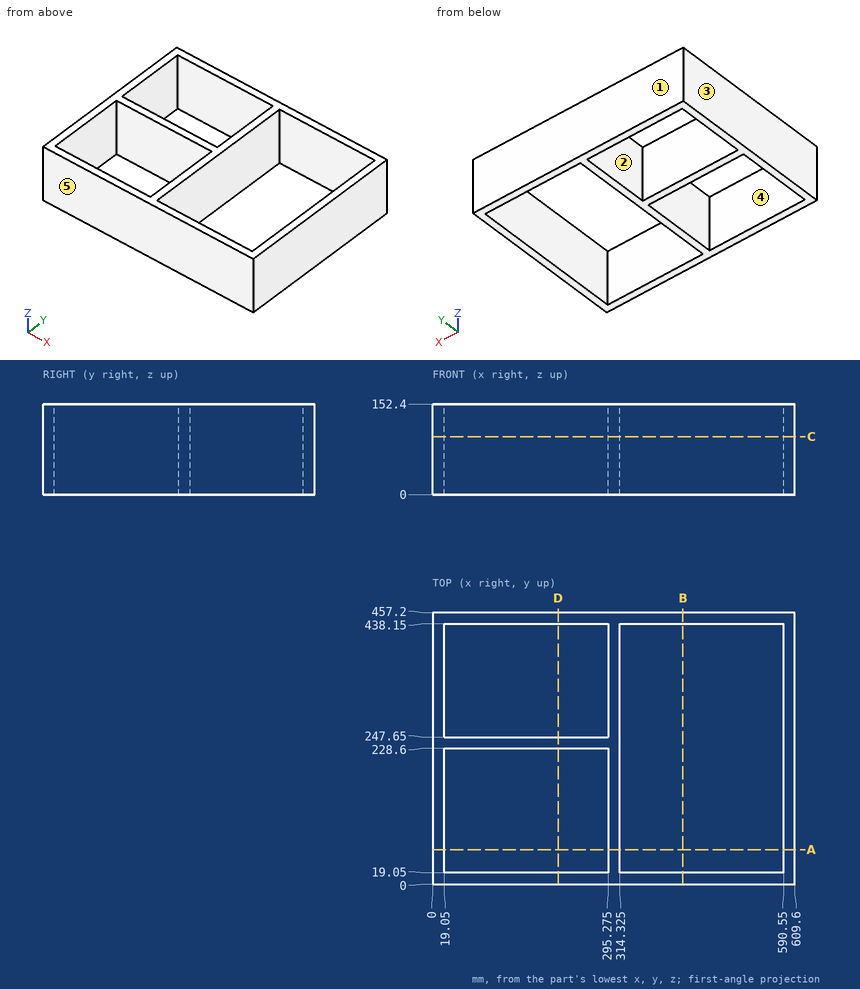
Answer from the drawing. Dimensions are ordinates in mm from the lowest x, y and z of the part. A direction names the side the tool comes from. Give positions to 0.01 mm unless a question says otherwise; leave off trailing zeros. Loops run counter-clockwise (first coordinate to the right, second up) from the corner with the lowest first, then second, coordinate; pieces in that order, holes last. Notation, with made-up numbers: (70, 68.25) - (108, 68.25) arc R24 ccw to (108, 78.25) - close; hole circle Ø9 at (30.25, -24.75). An arc over 180 degrees is marked (long way). Answer as CSV lines item,"result". Start each with the question number.
Item 1: Find the intervals of material crossed by line 1 (X direction, y = 334, z = 71.5) (3 decimals); line 2 (Y direction, x = 234.5, z = 42.5), in increasing order. Write a range as from..to.
Item 2: The mould has two halves that part along Y. Classify the marked faces 1, 2 and 3: +Y half, -Y half, draft (parallel to the pull), parting line (faces both ways), or undercut.
Item 3: A cutting plane is placed at B-B on x = 421. Determine the outline of the cut face in (y, z), then the cut area to 3 significant figures.
Item 4: A cutting plane is placed at D-D on x = 211. Determine the outline of the cut face in (y, z), then the cut area to 3 significant figures.
Item 5: A cutting plane is placed at A-A on y = 58.5. Determine the outline of the cut face in (x, z) (3 decimals), then the cut area to 3 significant figures.
Item 6: For the marked faces 4 and 5, determine the directions among +Z, -Z, +X, -X, +Y, -Y from which every point of the face is accessible in a straight line to the end or side of a thin tool.
Item 7: A cutting plane is placed at C-C on z = 97.5. Determine the outline of the cut face in (x, y) (3 decimals).
Found:
1,line 1,"x = 0..19.05, 295.275..314.325, 590.55..609.6"
1,line 2,"y = 0..19.05, 228.6..247.65, 438.15..457.2"
2,face 1,"+Y half"
2,face 2,"undercut"
2,face 3,"draft"
3,outline,"(0, 0) - (19.05, 0) - (19.05, 152.4) - (0, 152.4) - close; (438.15, 0) - (457.2, 0) - (457.2, 152.4) - (438.15, 152.4) - close"
3,area,"5,810 mm^2"
4,outline,"(0, 0) - (19.05, 0) - (19.05, 152.4) - (0, 152.4) - close; (228.6, 0) - (247.65, 0) - (247.65, 152.4) - (228.6, 152.4) - close; (438.15, 0) - (457.2, 0) - (457.2, 152.4) - (438.15, 152.4) - close"
4,area,"8,710 mm^2"
5,outline,"(0, 0) - (19.05, 0) - (19.05, 152.4) - (0, 152.4) - close; (295.275, 0) - (314.325, 0) - (314.325, 152.4) - (295.275, 152.4) - close; (590.55, 0) - (609.6, 0) - (609.6, 152.4) - (590.55, 152.4) - close"
5,area,"8,710 mm^2"
6,face 4,"+Z, -Z"
6,face 5,"+Z, -Z, +X, -X, -Y"
7,outline,"(0, 0) - (609.6, 0) - (609.6, 457.2) - (0, 457.2) - close; hole (19.05, 19.05) - (295.275, 19.05) - (295.275, 228.6) - (19.05, 228.6) - close; hole (19.05, 247.65) - (295.275, 247.65) - (295.275, 438.15) - (19.05, 438.15) - close; hole (314.325, 19.05) - (590.55, 19.05) - (590.55, 438.15) - (314.325, 438.15) - close"
